The figure shows three views and two pictorial views of one solid part (mm, origin at its lowest corner). Answer the questions. A direction names the side the tool comes from. Coordinates: 2 decimals unless noted, no trailing zeros. Write each loop counter-clockwise with the first axis right and the second up, starting at its lowest first coordinate (ties: lowest second). Pieces come first, ordered by that corner, then holes.
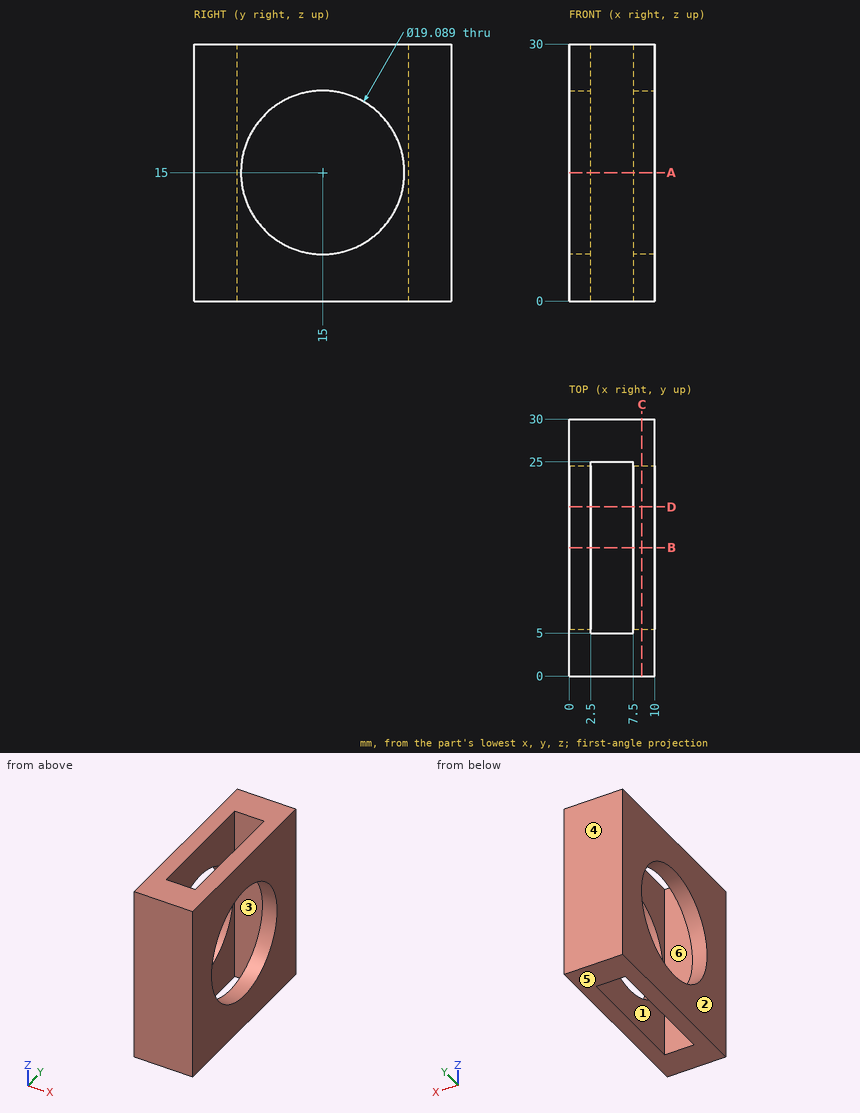
Q1. Find the intervals of material crossed by probe 1 along X at (y, z) = (16.5, 5.5); probe 2 along Y at (x, z) = (8.55, 15); probe 3 along Y at (x, z) = (7.25, 17), in increasing order.
Answers below:
probe 1: x = 0 to 2.5, 7.5 to 10
probe 2: y = 0 to 5.46, 24.54 to 30
probe 3: y = 0 to 5, 25 to 30
Q2. Determine the mould class of the marked faces 3, 4, 5 and 6 for opening direction Y: released by +Y, released by -Y, zero draft, split by the parting line, or undercut.
Answers below:
face 3: undercut
face 4: released by +Y
face 5: zero draft
face 6: undercut
Q3. The part is cut by section D-D, the plane y = 19.75. Write down the section's boundary in (x, z).
Answers below:
outline: (0, 0) - (2.5, 0) - (2.5, 6.72) - (0, 6.72) - close; (0, 23.28) - (2.5, 23.28) - (2.5, 30) - (0, 30) - close; (7.5, 0) - (10, 0) - (10, 6.72) - (7.5, 6.72) - close; (7.5, 23.28) - (10, 23.28) - (10, 30) - (7.5, 30) - close
Q4. The part is cut by section A-A, the plane z = 15. Write down the section's boundary in (x, y), then the cut area to 3 significant figures.
Answers below:
outline: (0, 0) - (10, 0) - (10, 5.46) - (7.5, 5.46) - (7.5, 5) - (2.5, 5) - (2.5, 5.46) - (0, 5.46) - close; (0, 24.54) - (2.5, 24.54) - (2.5, 25) - (7.5, 25) - (7.5, 24.54) - (10, 24.54) - (10, 30) - (0, 30) - close
area: 105 mm2
Q5. The part is cut by section C-C, the plane x = 8.5. Write down the section's boundary in (y, z), then the cut area to 3 significant figures.
Answers below:
outline: (0, 0) - (30, 0) - (30, 30) - (0, 30) - close; hole circle Ø19.09 at (15, 15)
area: 614 mm2
Q6. Given pin 1 (4 mm diameter, centred on x = 5, z = 10, fed in from -Y); pin 2 (15.5 mm diameter, centred on y = 15, z = 15, fed in from +X), each flat-ended and moving along its own axis, determine where each tip first touches the part or whether it passes through.
Answers below:
pin 1: stops at y = 0
pin 2: passes through
Q7. The part is cut by section B-B, the plane y = 15. Write down the section's boundary in (x, z).
Answers below:
outline: (0, 0) - (2.5, 0) - (2.5, 5.46) - (0, 5.46) - close; (0, 24.54) - (2.5, 24.54) - (2.5, 30) - (0, 30) - close; (7.5, 0) - (10, 0) - (10, 5.46) - (7.5, 5.46) - close; (7.5, 24.54) - (10, 24.54) - (10, 30) - (7.5, 30) - close
Q8. Which of the six approach directions +Z, -Z, +X, -X, +Y, -Y give full straight-line access (tool end or side, diameter ignored) to the marked faces 1 and 2?
Answers below:
face 1: +Z, -Z
face 2: +Z, -Z, -X, +Y, -Y
